```python
from build123d import *

# Parameters (mm, degrees)
F0_W     = 83.865903
F0_H     = 67.478316
F1_DEPTH = 50.8
F3_DEPTH = 74.422
F4_R     = 9.170677
F4_R_2   = 9.055805
F5_DEPTH = 65.278


with BuildPart() as f1:
    # F0 (on Front) → F1 (new body)
    with BuildSketch(Plane.XZ):
        with Locations((5.663358, -18.43604)):
            Rectangle(F0_W, F0_H)
    extrude(amount=F1_DEPTH)

    # F2 (on face) → F3 (cut)
    with BuildSketch(Plane.XY.offset(15.303118)):
        with BuildLine():
            ThreePointArc((-8.936779, 0), (5.663358, -14.600136), (20.263494, 0))
            Line((20.263494, 0), (-8.936779, 0))
        make_face()
    extrude(amount=-F3_DEPTH, mode=Mode.SUBTRACT)

    # F4 (on face) → F5 (cut)
    with BuildSketch(Plane(origin=(0, 0, 0), x_dir=(-1, 0, 0), z_dir=(0, 1, 0))):
        with Locations((26.124012, -23.695314)):
            Circle(F4_R)
        with Locations((-34.352176, -25.269844)):
            Circle(F4_R_2)
    extrude(amount=-F5_DEPTH, mode=Mode.SUBTRACT)


solid = f1.part
```
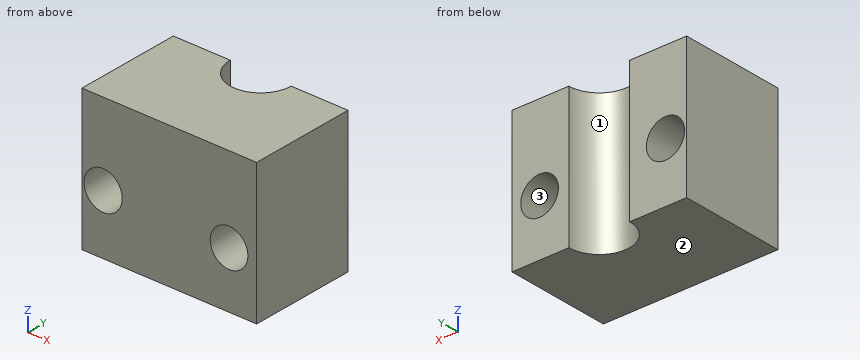
The listing builds one solid part. Answer for the finished solid, in the listing's coordinates (mm). Face numbers are marked on the shaded views. Give positions to 0.01 mm unless a question says otherwise; leave off trailing zeros. Loops run counter-clockwise (first coordinate to the right, second up) from the corner with the lowest first, then second, coordinate; pieces in that order, holes last. Notation, with made-up numbers: M 51,0.5 L 61,0.5 A8 cw 61,5.5 Z; hole C 19.25,60.5 d8. An arc over 180 degrees is marked long. One line per item, written item: value.
1. Find the intervals of material crossed by probe 1 along X at (y, z) = (-13.5, -15.5); probe 2 along X at (y, z) = (-46.5, -19.5); probe 3 along Y at (x, z) = (5, -14.5), in increasing order.
Found:
probe 1: -36.27 to -30.24, -22.01 to 0.1, 11.22 to 47.6
probe 2: -36.27 to -34.28, -17.97 to 27.37, 41.33 to 47.6
probe 3: -50.8 to -14.59
2. Section A-A on y = -10 is taken. Determine the outline of the cut face in (x, z).
Found:
outline: M -36.27,-52.18 L -4.97,-52.18 L -4.97,15.3 L -36.27,15.3 Z; M 16.3,-52.18 L 47.6,-52.18 L 47.6,15.3 L 16.3,15.3 Z; hole C -26.12,-23.7 d18.34; hole C 34.35,-25.27 d18.11
3. Section C-C on z = -42 is taken. Determine the outline of the cut face in (x, y), plus the area to 3 significant figures.
Found:
outline: M -36.27,-50.8 L 47.6,-50.8 L 47.6,0 L 20.26,0 A14.6 cw -8.94,0 L -36.27,0 Z
area: 3,930 mm^2
4. Section B-B on x = 30 is taken. Determine the outline of the cut face in (y, z), plus the area to 3 significant figures.
Found:
outline: M -50.8,-52.18 L 0,-52.18 L 0,-33.21 L -50.8,-33.21 Z; M -50.8,-17.33 L 0,-17.33 L 0,15.3 L -50.8,15.3 Z
area: 2,620 mm^2
5. This flat-tipped pin is pushed along its axis until it touches: P1, Ø1, axis at x = -17.5, z = 4.5, coming from the +Y side. Where does it stop, or does it pass through?
Found:
P1: y = 0
6. For a pull along Z with two mould halves and no side action, classify the marked faces 1, 2 and 3 as pulls with the +Z half, pulls with the -Z half, needs draft (parallel to the pull), parting line crosses it, or undercut.
Found:
face 1: needs draft
face 2: pulls with the -Z half
face 3: undercut
7. Section D-D on y = -16.5 is taken. Determine the outline of the cut face in (x, z).
Found:
outline: M -36.27,-52.18 L 47.6,-52.18 L 47.6,15.3 L -36.27,15.3 Z; hole C -26.12,-23.7 d18.34; hole C 34.35,-25.27 d18.11
